```python
from build123d import *

# Parameters (mm, degrees)
BOSS_EXTRUDE1_DEPTH = 12
SKETCH2_R           = 4
BOSS_EXTRUDE2_DEPTH = 6
SKETCH3_W           = 55.6
SKETCH3_H           = 2.5
BOSS_EXTRUDE3_DEPTH = 7
SKETCH5_W           = 3
SKETCH5_H           = 51.6
CUT_EXTRUDE1_DEPTH  = 42.791956142
FILLET3_R           = 2
CHAMFER1_SIZE       = 0.8
CHAMFER2_SIZE       = 0.8
CHAMFER3_SIZE       = 0.8


with BuildPart() as part:
    # Sketch1 → Boss-Extrude1 (new body)
    with BuildSketch(Plane(origin=(0, 0, 0), x_dir=(0, 0, -1), z_dir=(1, 0, 0))):
        Polygon((-29.89631037, 3.89631037), (-29.89631037, 1.39631037), (-35.89631037, 1.39631037), (-35.89631037, -1.20368963), (-29.89631037, -1.20368963), (-29.89631037, -2.45368963), (29.70368963, -2.45368963), (29.70368963, -1.20368963), (35.70368963, -1.20368963), (35.70368963, 1.39631037), (29.70368963, 1.39631037), (29.70368963, 3.89631037), align=None)
    extrude(amount=BOSS_EXTRUDE1_DEPTH)

    # Sketch2 → Boss-Extrude2 (add)
    with BuildSketch(Plane(origin=(0, 3.89631037, 0), x_dir=(1, 0, 0), z_dir=(0, 1, 0))):
        with Locations(Location((6, -20, 0), (0, 0, 90))):
            Circle(SKETCH2_R)
        with Locations(Location((6, 20, 0), (0, 0, 90))):
            Circle(SKETCH2_R)
    extrude(amount=BOSS_EXTRUDE2_DEPTH)

    # Sketch3 → Boss-Extrude3 (add)
    with BuildSketch(Plane(origin=(12, 0, 0), x_dir=(0, 0, -1), z_dir=(1, 0, 0))):
        with Locations((-0.09631037, -1.20368963)):
            Rectangle(SKETCH3_W, SKETCH3_H)
    extrude(amount=BOSS_EXTRUDE3_DEPTH)

    # Sketch5 → Cut-Extrude1 (cut, through all)
    with BuildSketch(Plane(origin=(0, 0.04631037, 0), x_dir=(1, 0, 0), z_dir=(0, 1, 0))):
        with Locations((15.5, -0.09631037)):
            Rectangle(SKETCH5_W, SKETCH5_H)
    extrude(amount=-CUT_EXTRUDE1_DEPTH, mode=Mode.SUBTRACT)

    # Fillet3
    fillet3_edges = [part.edges().sort_by_distance(p)[0] for p in [
        (19, -1.20368963, 27.89631037),
        (19, -1.20368963, -27.70368963),
    ]]
    fillet(fillet3_edges, radius=FILLET3_R)

    # Chamfer1
    chamfer1_edges = [part.edges().sort_by_distance(p)[0] for p in [
        (0, 2.64631037, -29.70368963),
        (0, 1.39631037, -32.70368963),
        (0, 0.09631037, -35.70368963),
        (0, -1.20368963, -32.70368963),
        (0, -1.82868963, -29.70368963),
        (0, -2.45368963, 0.09631037),
        (0, -1.82868963, 29.89631037),
        (0, -1.20368963, 32.89631037),
        (0, 0.09631037, 35.89631037),
        (0, 1.39631037, 32.89631037),
        (0, 2.64631037, 29.89631037),
        (0, 3.89631037, 0.09631037),
    ]]
    chamfer(chamfer1_edges, length=CHAMFER1_SIZE)

    # Chamfer2
    chamfer2_edges = [part.edges().sort_by_distance(p)[0] for p in [
        (6, 9.89631037, 24),
        (6, 9.89631037, -16),
    ]]
    chamfer(chamfer2_edges, length=CHAMFER2_SIZE)

    # Chamfer3
    chamfer3_edges = [part.edges().sort_by_distance(p)[0] for p in [
        (12, 1.39631037, 32.89631037),
        (12, 0.09631037, 35.89631037),
        (12, -1.20368963, 32.89631037),
        (12, -1.82868963, 29.89631037),
        (12, -2.45368963, 28.89631037),
        (12, -1.82868963, -29.70368963),
        (12, -1.20368963, -32.70368963),
        (12, 0.09631037, -35.70368963),
        (12, 1.39631037, -32.70368963),
        (12, -2.45368963, -28.70368963),
        (12, -1.20368963, 27.89631037),
        (12, -1.20368963, -27.70368963),
        (12, 2.64631037, -29.70368963),
        (12, 0.04631037, 0.09631037),
        (12, 3.89631037, 0.09631037),
        (15.5, 0.04631037, -25.70368963),
        (14, 0.04631037, 0.09631037),
        (15.5, 0.04631037, 25.89631037),
        (17, 0.04631037, 0.09631037),
        (19, -2.45368963, 0.09631037),
        (19, 0.04631037, 0.09631037),
        (14.5, 0.04631037, 27.89631037),
        (14.5, 0.04631037, -27.70368963),
        (18.414213562, 0.04631037, 27.310523932),
        (18.414213562, 0.04631037, -27.117903192),
        (14.5, -2.45368963, -27.70368963),
        (14.5, -2.45368963, 27.89631037),
        (18.414213562, -2.45368963, 27.310523932),
        (18.414213562, -2.45368963, -27.117903192),
        (12, 2.64631037, 29.89631037),
    ]]
    chamfer(chamfer3_edges, length=CHAMFER3_SIZE)


solid = part.part
```
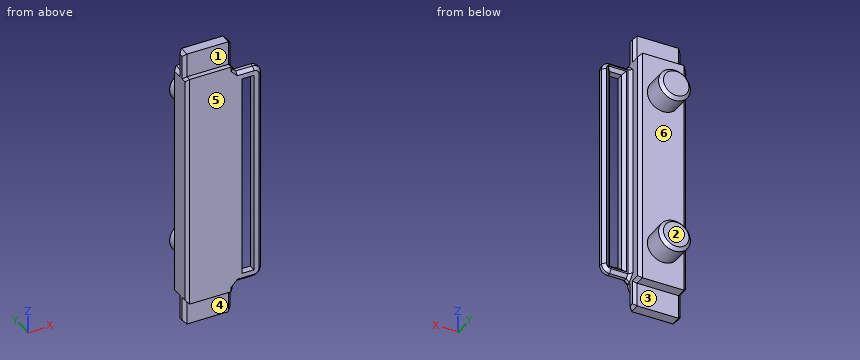
Model file for the job. Use its own axes, mm. Face numbers are marked on the shaded views. A direction names the side the tool comes from. Round coordinates to 2 decimals unless told otherwise and drop trailing zeros. Write each loop counter-clockwise with the first axis right and the second up, starting at its lowest first coordinate (ties: lowest second). Pieces come first, ordered by that corner, then holes. Notation, with made-up numbers: (3, 17.25) - (37, 17.25) arc R32 ccw to (37, 56.25) - close; hole circle Ø9 at (-25.75, 87). An arc over 180 degrees is marked (long way). One line per item, written item: value.
(1) Two-plate mould, pull along Z, no slides. Class the marked faces 5 and 6: pulls with the +Z half, pulls with the -Z half, needs draft (parallel to the pull), parting line crosses it, or undercut.
Values follow:
face 5: needs draft
face 6: undercut
(2) Cut at B-B, the plane x = 6. Give the cut face in (y, z), plus the area to 3 significant figures.
Values follow:
outline: (-2.45, -29.7) - (-1.2, -29.7) - (-1.2, -35.7) - (1.4, -35.7) - (1.4, -29.7) - (3.9, -29.7) - (3.9, -24) - (9.1, -24) - (9.9, -23.2) - (9.9, -16.8) - (9.1, -16) - (3.9, -16) - (3.9, 16) - (9.1, 16) - (9.9, 16.8) - (9.9, 23.2) - (9.1, 24) - (3.9, 24) - (3.9, 29.9) - (1.4, 29.9) - (1.4, 35.9) - (-1.2, 35.9) - (-1.2, 29.9) - (-2.45, 29.9) - close
area: 504 mm²
(3) Drop flat-ended pins along their axis: P1, Ø5, axis at x = 9.5, z = 0, coming from the +Y side; P2, Ø6, axis at y = 4, z = -11, coming from the +X side; P3, Ø3, axis at x = 4.5, y = 3, coming from the +Z side; P4, Ø2, axis at x = 12.5, y = 6, coming from the -Z side. Give the stop position or say it passes through.
Values follow:
P1: stops at y = 3.9
P2: stops at x = 12
P3: stops at z = 29.9
P4: passes through
(4) 3-axis set-ups, long thin cutter, end or side, ignore diameter. For the marked faces 1, 2, 3 and 4: which of +Z, -Z, +X, -X, +Y, -Y reach the whole face in a straight line?
Values follow:
face 1: +Z, +X, -X, -Y
face 2: +Z, -Z, +X, -X, +Y
face 3: -Z, +X, -X, +Y
face 4: -Z, +X, -X, -Y
(5) Cut at A-A, the plane z = -14.5. Give the cut face in (x, y).
Values follow:
outline: (0, -1.65) - (0.8, -2.45) - (14, -2.45) - (14, -0.75) - (13.2, 0.05) - (12.8, 0.05) - (12, 0.85) - (12, 3.1) - (11.2, 3.9) - (0.8, 3.9) - (0, 3.1) - close; (17, -2.45) - (18.2, -2.45) - (19, -1.65) - (19, -0.75) - (18.2, 0.05) - (17.8, 0.05) - (17, -0.75) - close
(6) Wall check: probe 1 along X at (y, z) = (-1, 23); probe 2 along Y at (x, z) = (3, 27.5); probe 3 along X at (y, z) = (-0.25, -31.5). Give the ranges that are in metal, low to high.
Values follow:
probe 1: x = 0 to 14, 17 to 19
probe 2: y = -2.45 to 3.9
probe 3: x = 0 to 12
(7) Cut at C-C, the plane y = 6.25. Give the cut face in (x, z).
Values follow:
outline: circle Ø8 at (6, -20); circle Ø8 at (6, 20)
